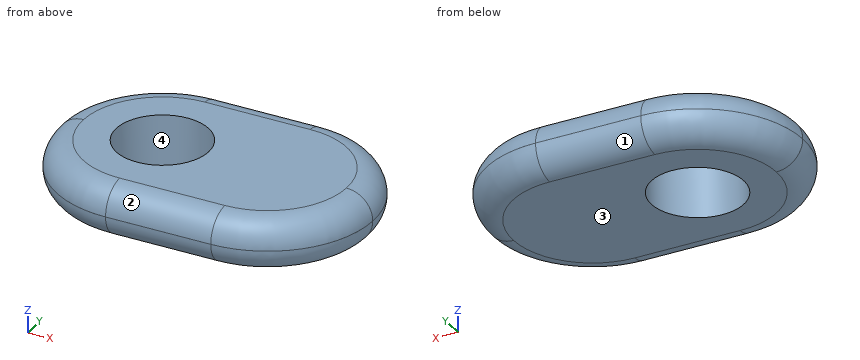
Autodesk Inventor part; units mm, degrees
ref_plane "YZ Plane" through (0, 0, 0) normal (1, 0, 0) x (0, 1, 0)
ref_plane "XZ Plane" through (0, 0, 0) normal (0, 1, 0) x (-1, 0, 0)
ref_plane "XY Plane" through (0, 0, 0) normal (0, 0, 1) x (1, 0, 0)
sketch "Sketch3" plane through (0, 0, 0) normal (0, 0, 1) x (1, 0, 0)
  line L0 (0, 0) -> (12, 0)
  line L1 (12, 0) -> (12, 8)
  line L2 (12, 8) -> (0, 8)
  line L3 (0, 8) -> (0, 0)
  dimension "d6" = 12
  dimension "d7" = 8
extrude "Extrusion2" add sketch "Sketch3" along normal blind 2
fillet "Fillet2" radius 4 4 edges at (0, 8, 1) (0, 0, 1) (12, 0, 1) (12, 8, 1)
sketch "Sketch4" plane through (0, 0, 2) normal (0, 0, 1) x (1, 0, 0)
  arc A0 (4, 8) -> (4, 0) centre (4, 4) ccw
  circle A1 centre (4, 4) radius 1.75
  point P0 (0, 0)
  dimension "d11" = 3.5
extrude "Extrusion3" cut sketch "Sketch4" against normal blind 2
fillet "Fillet3" radius 1 8 edges at (1.1714, 6.8286, 2) (6, 0, 2) (10.8286, 1.1714, 2) (6, 8, 2) (1.1714, 6.8286, 0) (6, 0, 0) (10.8286, 1.1714, 0) (6, 8, 0)
properties part number "Plectrum"
For this review, take the finished solid that the model builds, in its own axes (mm). Face numbers are marked on the shaded views. Round coordinates to 2 decimals unless told otherwise and drop trailing zeros. Answer as CSV lines item,"result".
(1) Wall thickness on line 1 (Y direction, x = 4, z = 0.85); line 2 (X direction, y = 5.5, z = 1.2); line 3 (X direction, y = 3, z = 1.3): over which ranges is each line inside the solid? List them lowest first.
Checked values:
line 1,"y = 0.01 to 2.25, 5.75 to 7.99"
line 2,"x = 0.31 to 3.1, 4.9 to 11.69"
line 3,"x = 0.17 to 2.56, 5.44 to 11.83"
(2) Mouldability with a two-part tool opening along Y and no side actions: class the marked faces 1, 2, 3 and 4 as +Y half, -Y half, draft (parallel to the pull), parting line (faces both ways), or undercut.
Checked values:
face 1,"+Y half"
face 2,"-Y half"
face 3,"draft"
face 4,"undercut"
(3) Insertion check: P1, Ø1, axis at x = 1.5, z = 2, coming from the -Y side. The pin has a flat end and moves straight along its axis. Give the tip position at first contact, or say it passes through.
Checked values:
P1,"stops at y = 0.9"
